For this review, take the finished solid that the model builds, in its own axes (mm). Face numbers are marked on the shaded views. A direction names the side the tool comes from. Give positions to 0.01 mm unless a question says otherwise; leave off trailing zeros. Order: outer loops, then holes, each group sorted by start corner. A loop starts at its lowest first (then second) coordinate and runs counter-clockwise, first axis right, second up. Notation, with made-up numbers: M 66,48 L 112,48 A10 cw 112,52 Z; hole C -3,36.5 d11. An arc over 180 degrees is marked long. Use CSV: the item, a comma, the result in double quotes. Start each with the question number.
(1) Tool access review of the marked faces 1 and 2: name each direction out of +Z, -Z, +X, -X, +Y, -Y from which nothing blocks a thin tool from reaching the whole face with its end or side.
(2) Consider section B-B (x = 21). Write out the cut boundary in (y, z), and give its area (3 significant figures).
(3) Consider section A-A (z = -21). Write out the cut boundary in (x, y), and give its area (3 significant figures).
(4) Consider section C-C (y = 15). Write out the cut boundary in (x, z), and give its area (3 significant figures).
(5) Wall thickness on L1, parallel to Y at x = 1, z = -21; L2, parallel to Z at x = 17, y = 94.5; L3, parallel to X at y = 49.5, z = -36: over which ranges is each line inside the solid? List them lowest first. Write a range as from..to.
(6) Consider section D-D (y = 175.5). Write out the cut boundary in (x, z), and give its area (3 significant figures).
(7) Clearance check with flat-ended pins moving along their axes: P1, Ø6, axis at y = 155, z = -30.5, coming from the +X side; P2, Ø3, axis at x = 34.5, y = 70, coming from the -Z side. State where each tip first meets the part, or that it passes through.
```python
from build123d import *

# Parameters (mm, degrees)
EXTRUDE_1_DEPTH     = 210
SKETCH_2_R          = 5
CUT_EXTRUDE_1_DEPTH = 41
SKETCH_3_R          = 5
CUT_EXTRUDE_2_DEPTH = 41


with BuildPart() as part:
    # Эскиз1 → Вытянуть-Тонкостенный1 (new body)
    with BuildSketch(Plane(origin=(0, 0, 0), x_dir=(1, 0, 0), z_dir=(0, 1, 0))):
        Polygon((0, 40), (0, 0), (40, 0), (40, 3), (3, 3), (3, 40), align=None)
    extrude(amount=EXTRUDE_1_DEPTH)

    # Эскиз2 → Вырез-Вытянуть1 (cut, through all)
    with BuildSketch(Plane.ZY):
        with Locations((-21, 15)):
            Circle(SKETCH_2_R)
        with Locations((-21, 75)):
            Circle(SKETCH_2_R)
        with Locations((-21, 135)):
            Circle(SKETCH_2_R)
        with Locations((-21, 195)):
            Circle(SKETCH_2_R)
    extrude(amount=-CUT_EXTRUDE_1_DEPTH, mode=Mode.SUBTRACT)

    # Эскиз3 → Вырез-Вытянуть2 (cut, through all)
    with BuildSketch(Plane.XY):
        with Locations((21, 15)):
            Circle(SKETCH_3_R)
        with Locations((21, 75)):
            Circle(SKETCH_3_R)
        with Locations((21, 135)):
            Circle(SKETCH_3_R)
        with Locations((21, 195)):
            Circle(SKETCH_3_R)
    extrude(amount=-CUT_EXTRUDE_2_DEPTH, mode=Mode.SUBTRACT)


solid = part.part
```
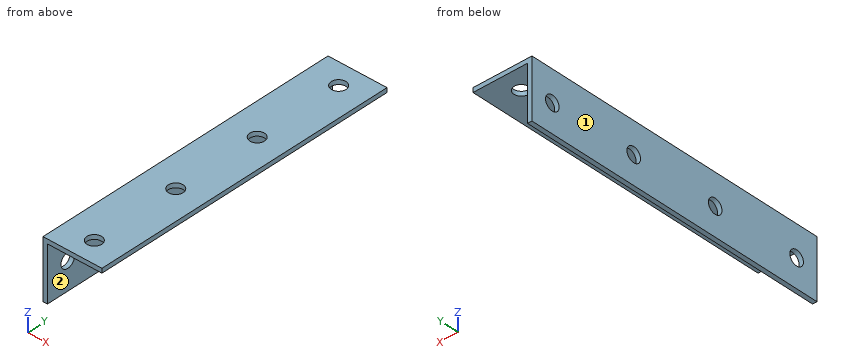
Check result:
1,face 1,"+Z, -Z, -X, +Y, -Y"
1,face 2,"-Z, +X, +Y, -Y"
2,outline,"M 0,-3 L 10,-3 L 10,0 L 0,0 Z; M 20,-3 L 70,-3 L 70,0 L 20,0 Z; M 80,-3 L 130,-3 L 130,0 L 80,0 Z; M 140,-3 L 190,-3 L 190,0 L 140,0 Z; M 200,-3 L 210,-3 L 210,0 L 200,0 Z"
2,area,"510 mm^2"
3,outline,"M 0,0 L 3,0 L 3,10 L 0,10 Z; M 0,20 L 3,20 L 3,70 L 0,70 Z; M 0,80 L 3,80 L 3,130 L 0,130 Z; M 0,140 L 3,140 L 3,190 L 0,190 Z; M 0,200 L 3,200 L 3,210 L 0,210 Z"
3,area,"510 mm^2"
4,outline,"M 0,-40 L 3,-40 L 3,-26 L 0,-26 Z; M 0,-16 L 3,-16 L 3,-3 L 16,-3 L 16,0 L 0,0 Z; M 26,-3 L 40,-3 L 40,0 L 26,0 Z"
4,area,"171 mm^2"
5,L1,"y = 0..10, 20..70, 80..130, 140..190, 200..210"
5,L2,"z = -3..0"
5,L3,"x = 0..3"
6,outline,"M 0,-40 L 3,-40 L 3,-3 L 40,-3 L 40,0 L 0,0 Z"
6,area,"231 mm^2"
7,P1,"stops at x = 3"
7,P2,"stops at z = -3"
